from build123d import *

# Parameters (mm, degrees)
SKETCH1_W                       = 60.458144771
SKETCH1_H                       = 61.20911147
BOSS_EXTRUDE1_DEPTH             = 3.175
F_1_4_0_25_DIAMETER_HOLE1_D     = 6.35
F_1_4_0_25_DIAMETER_HOLE1_DEPTH = 9.268267535
F_1_4_0_25_DIAMETER_HOLE1_TIP   = 1.907732465
CUT_EXTRUDE1_DEPTH              = 46.980601635
FILLET1_R                       = 12.7


with BuildPart() as part:
    # Sketch1 → Boss-Extrude1 (new body)
    with BuildSketch(Plane.XY):
        with Locations((3.939572159, 0)):
            Rectangle(SKETCH1_W, SKETCH1_H)
    extrude(amount=BOSS_EXTRUDE1_DEPTH)

    # 1/4 (0.25) Diameter Hole1
    with Locations(Plane.XY.offset(3.175)):
        with Locations((-0.282440227, 15.955359735)):
            Hole(F_1_4_0_25_DIAMETER_HOLE1_D / 2, depth=F_1_4_0_25_DIAMETER_HOLE1_DEPTH)
            with Locations((0, 0, -(F_1_4_0_25_DIAMETER_HOLE1_DEPTH + F_1_4_0_25_DIAMETER_HOLE1_TIP / 2))):  # 118° drill point
                Cone(0, F_1_4_0_25_DIAMETER_HOLE1_D / 2, F_1_4_0_25_DIAMETER_HOLE1_TIP, mode=Mode.SUBTRACT)

    # Sketch4 → Cut-Extrude1 (cut, through all)
    with BuildSketch(Plane(origin=(0, 0, 0), x_dir=(-1, 0, 0), z_dir=(0, 0, -1))):
        Polygon((26.289500227, -1.224692265), (-8.635499773, 8.379555735), (-8.635499773, 30.604555735), (-34.168644544, 30.604555735), (-34.168644544, -30.604555735), (26.289500227, -30.604555735), align=None)
    extrude(amount=-CUT_EXTRUDE1_DEPTH, mode=Mode.SUBTRACT)

    # Fillet1
    # the kernel refuses this fillet: 12.7 mm, written as the material it takes off along each edge
    with BuildSketch(Plane(origin=(8.635499773, 30.604555735, -31.75), x_dir=(-1, 0, 0), z_dir=(0, 0, 1))) as fillet1_piece_1:
        with BuildLine():
            CenterArc((FILLET1_R, FILLET1_R), FILLET1_R, 180, 90)
            Line((0, FILLET1_R), (0, 0))
            Line((0, 0), (FILLET1_R, 0))
        make_face()
    extrude(amount=66.675, mode=Mode.SUBTRACT)
    with BuildSketch(Plane(origin=(8.635499773, 8.379555735, -24.197503605), x_dir=(0, 1, 0), z_dir=(0, 0, 1))) as fillet1_piece_2:
        with BuildLine():
            CenterArc((FILLET1_R * 0.762126097799, FILLET1_R), FILLET1_R, 195.376057549, 74.623942451)
            Line((-FILLET1_R * 0.202080191414, FILLET1_R * 0.734846776671), (0, 0))
            Line((0, 0), (FILLET1_R * 0.762126097799, 0))
        make_face()
    extrude(amount=51.57000721, mode=Mode.SUBTRACT)


solid = part.part
For this review, take the finished solid that the model builds, in its own axes (mm). Round coordinates to 2 decimals unless told otherwise and drop trailing zeros. Order: outer loops, then holes, each group sorted by start corner. A loop starts at its lowest first (then second) coordinate and runs counter-clockwise, first axis right, second up. Notation, with made-up numbers: (58, 79.5) -> (108, 79.5) arc R22 cw to (108, 99.5) -> close; hole circle Ø11 at (-16.75, 69). An arc over 180 degrees is marked (long way). Write item = value, one per line. Start each with the question number.
1) Take a section at A-A on y = 17. State the section outline as (x, z) points (1 decimal).
2) Insertion check: pin 1 (1.5 mm diameter, centred on x = -1.5, y = 4.5, fed in from +Z). The pin has a flat end and moves straight along its axis. Give the tip position at first contact, or say it passes through.
3) Take a section at D-D on y = 27. State the section outline as (x, z) points (1 decimal).
4) To check wall thickness, follow line 1 (Y direction, x = -1.5, z = 2.9); line 2 (Y direction, x = 2, z = 2.6); line 3 (X direction, y = 14, z = 1.25). State the ranges of each line that lie inside material, in increasing order. Write a range as from..to.
5) The part is to be moulded in two halves that separate along X. For faces 1 (the face through (-26.29, 14, 2)), 2 (the face through (0.406, 12.856, 1.565)), 3 (the face through (-13.672, 2.245, 1.565)), 4 (the face through (-13, 15, 0)), say which applies: +X half, -X half, draft (parallel to the pull), parting line (faces both ways), or undercut.
6) Take a section at C-C on x = 6. State the section outline as (y, z) points (3 decimals).
Verdict:
q1.outline = (-26.3, 0) -> (-3.3, 0) -> (-3.3, 3.2) -> (-26.3, 3.2) -> close; (2.7, 0) -> (8.6, 0) -> (8.6, 3.2) -> (2.7, 3.2) -> close
q2.pin_1 = through
q3.outline = (-26.3, 0) -> (4.8, 0) -> (4.8, 3.2) -> (-26.3, 3.2) -> close
q4.line_1 = 5.59..13.02, 18.89..30.34
q4.line_2 = 6.9..13.75, 18.16..29.06
q4.line_3 = -26.29..-2.78, 2.22..7.97
q5.face_1 = -X half
q5.face_2 = undercut
q5.face_3 = +X half
q5.face_4 = draft
q6.outline = (10.313, 0) -> (25.65, 0) -> (25.65, 3.175) -> (10.313, 3.175) -> close
